```python
from build123d import *
from build123d.topology import SkipClean

# Parameters (mm, degrees)
SKETCH_1_R          = 21
EXTRUDE_1_DEPTH     = 15
EXTRUDE_START       = 6
EXTRUDE_2_DEPTH     = 6
EXTRUDE_3_DEPTH     = 6
EXTRUDE_START_2     = 9
EXTRUDE_4_DEPTH     = 9
SKETCH_6_R          = 7.5
EXTRUDE_5_DEPTH     = 1
SKETCH_7_R          = 3
EXTRUDE_6_DEPTH     = 15
SKETCH_8_R          = 1.5
CUT_EXTRUDE_1_DEPTH = 3


with BuildPart() as part:
    # 草图1 → 凸台-拉伸1 (new body)
    with BuildSketch(Plane.XY):
        Circle(SKETCH_1_R)
    extrude(amount=EXTRUDE_1_DEPTH)

    # 草图2 → 凸台-拉伸2 (add)
    with SkipClean():  # the faces are left unmerged after this step: merging them gives an invalid solid
        with BuildSketch(Plane(origin=(0, 0, 0), x_dir=(-1, 0, 0), z_dir=(0, 0, -1)).offset(EXTRUDE_START)):
            with BuildLine():
                Line((2.5, 20.850659462), (2.5, 20.346989949))
                ThreePointArc((2.5, 20.346989949), (0, 20.5), (-2.5, 20.346989949))
                Line((-2.5, 20.346989949), (-2.5, 20.850659462))
                ThreePointArc((-2.5, 20.850659462), (-18.186533479, 10.5), (-19.30720078, -8.260266222))
                Line((-19.30720078, -8.260266222), (-18.871010187, -8.008431465))
                ThreePointArc((-18.871010187, -8.008431465), (-17.753520778, -10.25), (-16.371010187, -12.338558484))
                Line((-16.371010187, -12.338558484), (-16.80720078, -12.59039324))
                ThreePointArc((-16.80720078, -12.59039324), (-15.938440593, -13.673555187), (-15, -14.696938457))
                Line((-15, -14.696938457), (-15, -13.973188612))
                ThreePointArc((-15, -13.973188612), (0, -20.5), (15, -13.973188612))
                Line((15, -13.973188612), (15, -14.696938457))
                ThreePointArc((15, -14.696938457), (15.938440593, -13.673555187), (16.80720078, -12.59039324))
                Line((16.80720078, -12.59039324), (16.371010187, -12.338558484))
                ThreePointArc((16.371010187, -12.338558484), (17.753520778, -10.25), (18.871010187, -8.008431465))
                Line((18.871010187, -8.008431465), (19.30720078, -8.260266222))
                ThreePointArc((19.30720078, -8.260266222), (18.186533479, 10.5), (2.5, 20.850659462))
            make_face()
        extrude(amount=-EXTRUDE_2_DEPTH)

    # 草图4 → 凸台-拉伸3 (add)
    with SkipClean():  # the faces are left unmerged after this step: merging them gives an invalid solid
        with BuildSketch(Plane(origin=(0, 0, -6), x_dir=(-1, 0, 0), z_dir=(0, 0, -1)).offset(EXTRUDE_START)):
            with BuildLine():
                Line((10, -17.895530168), (10, -24))
                Line((10, -24), (-10, -24))
                Line((-10, -24), (-10, -17.895530168))
                ThreePointArc((-10, -17.895530168), (-12.652912345, -16.129284212), (-15, -13.973188612))
                Line((-15, -13.973188612), (-15, -14.696938457))
                ThreePointArc((-15, -14.696938457), (-15.938440593, -13.673555187), (-16.80720078, -12.59039324))
                Line((-16.80720078, -12.59039324), (-16.371010187, -12.338558484))
                ThreePointArc((-16.371010187, -12.338558484), (-17.753520778, -10.25), (-18.871010187, -8.008431465))
                Line((-18.871010187, -8.008431465), (-19.30720078, -8.260266222))
                ThreePointArc((-19.30720078, -8.260266222), (-18.186533479, 10.5), (-2.5, 20.850659462))
                Line((-2.5, 20.850659462), (-2.5, 20.346989949))
                ThreePointArc((-2.5, 20.346989949), (0, 20.5), (2.5, 20.346989949))
                Line((2.5, 20.346989949), (2.5, 20.850659462))
                ThreePointArc((2.5, 20.850659462), (18.186533479, 10.5), (19.30720078, -8.260266222))
                Line((19.30720078, -8.260266222), (18.871010187, -8.008431465))
                ThreePointArc((18.871010187, -8.008431465), (17.753520778, -10.25), (16.371010187, -12.338558484))
                Line((16.371010187, -12.338558484), (16.80720078, -12.59039324))
                ThreePointArc((16.80720078, -12.59039324), (15.938440593, -13.673555187), (15, -14.696938457))
                Line((15, -14.696938457), (15, -13.973188612))
                ThreePointArc((15, -13.973188612), (12.652912345, -16.129284212), (10, -17.895530168))
            make_face()
        extrude(amount=-EXTRUDE_3_DEPTH)

    # 草图5 → 凸台-拉伸4 (add)
    with SkipClean():  # the faces are left unmerged after this step: merging them gives an invalid solid
        with BuildSketch(Plane(origin=(0, 0, -12), x_dir=(-1, 0, 0), z_dir=(0, 0, -1)).offset(EXTRUDE_START_2)):
            with BuildLine():
                Line((18.871010187, -8.008431465), (19.30720078, -8.260266222))
                ThreePointArc((19.30720078, -8.260266222), (18.186533479, 10.5), (2.5, 20.850659462))
                Line((2.5, 20.850659462), (2.5, 20.346989949))
                ThreePointArc((2.5, 20.346989949), (0, 20.5), (-2.5, 20.346989949))
                Line((-2.5, 20.346989949), (-2.5, 20.850659462))
                ThreePointArc((-2.5, 20.850659462), (-18.186533479, 10.5), (-19.30720078, -8.260266222))
                Line((-19.30720078, -8.260266222), (-18.871010187, -8.008431465))
                ThreePointArc((-18.871010187, -8.008431465), (-17.753520778, -10.25), (-16.371010187, -12.338558484))
                Line((-16.371010187, -12.338558484), (-16.80720078, -12.59039324))
                ThreePointArc((-16.80720078, -12.59039324), (-15.938440593, -13.673555187), (-15, -14.696938457))
                ThreePointArc((-15, -14.696938457), (0, -21), (15, -14.696938457))
                ThreePointArc((15, -14.696938457), (15.938440593, -13.673555187), (16.80720078, -12.59039324))
                Line((16.80720078, -12.59039324), (16.371010187, -12.338558484))
                ThreePointArc((16.371010187, -12.338558484), (17.753520778, -10.25), (18.871010187, -8.008431465))
            make_face()
        extrude(amount=-EXTRUDE_4_DEPTH)

    # 草图6 → 凸台-拉伸5 (add)
    with SkipClean():  # the faces are left unmerged after this step: merging them gives an invalid solid
        with BuildSketch(Plane.XY.offset(15)):
            Circle(SKETCH_6_R)
        extrude(amount=EXTRUDE_5_DEPTH)

    # 草图7 → 凸台-拉伸6 (add)
    with SkipClean():  # the faces are left unmerged after this step: merging them gives an invalid solid
        with BuildSketch(Plane.XY.offset(16)):
            Circle(SKETCH_7_R)
        extrude(amount=EXTRUDE_6_DEPTH)

    # 草图8 → 切除-拉伸1 (cut)
    with SkipClean():  # the faces are left unmerged after this step: merging them gives an invalid solid
        with BuildSketch(Plane.XY.offset(15)):
            with Locations((0, 15.5)):
                Circle(SKETCH_8_R)
            with Locations((13.12709029, 8.241935484)):
                Circle(SKETCH_8_R)
            with Locations((13.960339517, -6.734903159)):
                Circle(SKETCH_8_R)
            with Locations((-13.12709029, -8.241935484)):
                Circle(SKETCH_8_R)
        extrude(amount=-CUT_EXTRUDE_1_DEPTH, mode=Mode.SUBTRACT)


solid = part.part
```
Verification items for the finished model (mm, model axes). A direction names the side the tool comes from. Coordinates: 2 decimals unless noted, no trailing zeros. Write each loop counter-clockwise with the first axis right and the second up, starting at its lowest first coordinate (ties: lowest second). Pieces come first, ordered by that corner, then holes. Notation, with made-up numbers: M -26.5,-15 L -11.5,-15 A14 cw -11.5,7 Z; hole C -22.75,28 d5. An arc over 180 degrees is marked long. Answer as a JSON object with one key per item and string values. Group by question number.
(1) Release check for a two-part mould opening along X. For faces 1 (the face through (10, -21, -9)), 2 (the face through (-3, 0, 23)), 3 (the face through (-13, -8, 12)), 4 (the face through (0, -22, -12)) record: +X half, -X half, draft (parallel to the pull), parting line (faces both ways), or undercut.
(2) Tool access check on faces 5 (the face through (0, -24, -9)), 6 (the face through (14.513, 7.667, 13.521)). Record the directions out of +Z, -Z, +X, -X, +Y, -Y that give a thin tool (end or side, any length) a straight path to the whole face; none if there is none.
(3) Cross-section at C-C, the plane y = 0. Record the cut outline in (x, z).
(4) Cross-section at B-B, the plane x = 0. Record the cut outline in (y, z).
(5) Cross-section at D-D, the plane z = -8. Record the cut outline in (x, y), and give its area (3 significant figures).
(6) Material ranges on line 1 (Z direction, x = -10, y = 0.5); line 2 (Y direction, x = 0, z = 14); line 3 (Y direction, x = -16.5, z = -14.5), recorded low to high.
(7) Cross-section at A-A, the plane z = -15.5. Record the cut outline in (x, y).
(8) Gauge pin test, flat ends, axial feed: pin 1 (3.5 mm diameter, centred on x = -12, y = -16, fed in from +Z); pin 2 (1.5 mm diameter, centred on x = -1, y = -4, fed in from +Z); pin 3 (10 mm diameter, centred on y = -3, z = -8.5, fed in from -X). Record the tip position at first contact, or that the pin passes through.
Reply:
{
 "1": {"face 1": "+X half", "face 2": "parting line", "face 3": "undercut", "face 4": "draft"},
 "2": {"face 5": "+Z, -Z, +X, -X, -Y", "face 6": "+Z"},
 "3": {"outline": "M -21,-21 L 21,-21 L 21,15 L 7.5,15 L 7.5,16 L 3,16 L 3,31 L -3,31 L -3,16 L -7.5,16 L -7.5,15 L -21,15 Z"},
 "4": {"outline": "M -24,-12 L -21,-12 L -21,-21 L 20.5,-21 L 20.5,0 L 21,0 L 21,15 L 17,15 L 17,12 L 14,12 L 14,15 L 7.5,15 L 7.5,16 L 3,16 L 3,31 L -3,31 L -3,16 L -7.5,16 L -7.5,15 L -21,15 L -21,0 L -20.5,0 L -20.5,-6 L -24,-6 Z"},
 "5": {"outline": "M -19.31,-8.26 L -18.87,-8.01 A20.5 ccw -16.37,-12.34 L -16.81,-12.59 A21 ccw -15,-14.7 L -15,-13.97 A20.5 ccw -10,-17.9 L -10,-24 L 10,-24 L 10,-17.9 A20.5 ccw 15,-13.97 L 15,-14.7 A21 ccw 16.81,-12.59 L 16.37,-12.34 A20.5 ccw 18.87,-8.01 L 19.31,-8.26 A21 ccw 2.5,20.85 L 2.5,20.35 A20.5 ccw -2.5,20.35 L -2.5,20.85 A21 ccw Z", "area": "1,450 mm²"},
 "6": {"line 1": "-21 to 15", "line 2": "-21 to 14, 17 to 21", "line 3": "-12.99 to -12.41, -12.17 to 12.99"},
 "7": {"outline": "M -19.31,-8.26 L -18.87,-8.01 A20.5 ccw -16.37,-12.34 L -16.81,-12.59 A21 ccw 16.81,-12.59 L 16.37,-12.34 A20.5 ccw 18.87,-8.01 L 19.31,-8.26 A21 ccw 2.5,20.85 L 2.5,20.35 A20.5 ccw -2.5,20.35 L -2.5,20.85 A21 ccw Z"},
 "8": {"pin 1": "z = 15", "pin 2": "z = 16", "pin 3": "x = -21"}
}
